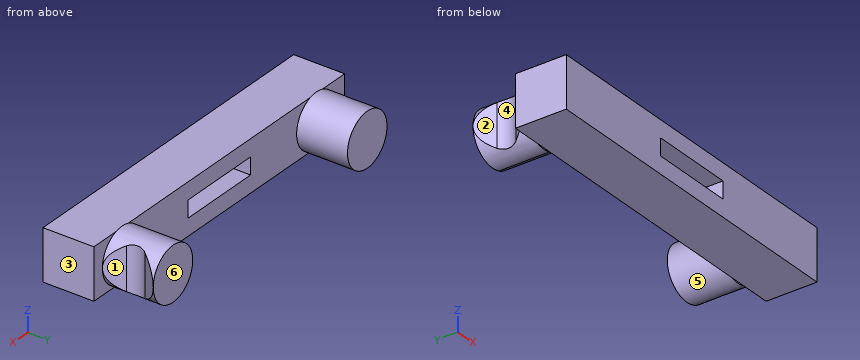
from build123d import *
from build123d.topology import SkipClean

# Parameters (mm, degrees)
SKETCH1_W            = 50.8
SKETCH1_H            = 7.62
BOSS_EXTRUDE1_DEPTH  = 7.62
SKETCH2_W            = 12.7
SKETCH2_H            = 2.54
CUT_EXTRUDE1_DEPTH   = 27.790679349
SKETCH3_R            = 4
BOSS_EXTRUDE2_DEPTH  = 7.62
CUT_EXTRUDE2_DEPTH   = 7.62
FILLET1_R            = 2.54
FILLET1_OF_MIRROR1_R = 2.54


with BuildPart() as part:
    # Sketch1 → Boss-Extrude1 (new body)
    with BuildSketch(Plane(origin=(0, 0, 0), x_dir=(1, 0, 0), z_dir=(0, 1, 0))):
        Rectangle(SKETCH1_W, SKETCH1_H)
    extrude(amount=BOSS_EXTRUDE1_DEPTH)

    # Sketch2 → Cut-Extrude1 (cut, through all)
    with BuildSketch(Plane(origin=(0, 7.62, 0), x_dir=(1, 0, 0), z_dir=(0, 1, 0))):
        Rectangle(SKETCH2_W, SKETCH2_H)
    extrude(amount=-CUT_EXTRUDE1_DEPTH, mode=Mode.SUBTRACT)

    # Sketch3 → Boss-Extrude2 (add)
    with BuildSketch(Plane(origin=(0, 7.62, 0), x_dir=(1, 0, 0), z_dir=(0, 1, 0))):
        with Locations(Location((-19.681240592, 0, 0), (0, 0, 72.269593739))):
            Circle(SKETCH3_R)
    boss_extrude2 = extrude(amount=BOSS_EXTRUDE2_DEPTH)

    # Sketch4 → Cut-Extrude2 (cut, symmetric)
    with SkipClean():  # the faces are left unmerged after this step: merging them gives an invalid solid
        with BuildSketch(Plane.XY):
            Polygon((-23.681240592, 15.24), (-23.681240592, 7.62), (-21.141240592, 11.43), align=None)
        cut_extrude2 = extrude(amount=CUT_EXTRUDE2_DEPTH, both=True, mode=Mode.SUBTRACT)

    # Fillet1
    fillet1_edges = [part.edges().sort_by_distance(p)[0] for p in [
        (-21.141240592, 11.43, 0),
    ]]
    fillet(fillet1_edges, radius=FILLET1_R)

    # Mirror1: Boss-Extrude2, Cut-Extrude2 across plane
    add(boss_extrude2.mirror(Plane(origin=(0, 0, 0), x_dir=(0, 0, 1), z_dir=(1, 0, 0))))
    add(cut_extrude2.mirror(Plane(origin=(0, 0, 0), x_dir=(0, 0, 1), z_dir=(1, 0, 0))), mode=Mode.SUBTRACT)

    # Fillet1 of Mirror1
    fillet1_of_mirror1_edges = [part.edges().sort_by_distance(p)[0] for p in [
        (21.141240592, 11.43, 0),
    ]]
    fillet(fillet1_of_mirror1_edges, radius=FILLET1_OF_MIRROR1_R)


solid = part.part
Can you work these out from the model? Positions are in its coordinate system, mm. Face numbers are marked on the shaded views. A direction names the side the tool comes from. Coordinates: 2 decimals unless noted, no trailing zeros. Loops run counter-clockwise (first coordinate to the right, second up) from the corner with the lowest first, then second, coordinate; pieces in that order, holes last. Notation, with made-up numbers: M -15,-31.75 L 5,-31.75 A28 cw 5,1.25 Z; hole C -27,-27.5 d8. An arc over 180 degrees is marked long. Answer as CSV lines item,"result". Start each with the question number.
1. For pin 1 Ø2.5 at (x, z) = (7.5, 2) entering from +Y; pin 2 Ø2 at (x, z) = (-16.5, 2.5) entering from +Y; pin 3 Ø2.5 at (x, y) = (2, 3.5) entering from +Z; pin 4 Ø6 at (x, y) = (-1, 3.5) entering from -Z, each with a flat end and sliding along its axis, tell me the tip position at first contact or that it passes through.
2. Suppose I cut it at C-C, the plane z = 0.5. List the corners of the cut face in (x, y) for me, plus the area to 3 significant figures.
3. Suppose I cut it at B-B, the plane y = 7. List the corners of the cut face in (x, z) for me.
4. Suppose I cut it at A-A, the plane x = -3. List the corners of the cut face in (y, z) for me, plus the area to 3 significant figures.
5. If I drill on probe 1 along Z at (x, y) = (-3, 4.5); probe 2 along X at (y, z) = (3.5, -0.25); probe 3 along Y at (x, z) = (-2, -2.25), over which ranges is the centre line in solid material (lowest first)? Write a range as [from, to].
6. Thinking about a two-plate mould opening in X: for the marked faces 4, 5 and 6, which applies, +X half, -X half, draft (parallel to the pull), parting line (faces both ways), or undercut?
7. Suppose I cut it at D-D, the plane y = 9. List the corners of the cut face in (x, z) for me, plus the area to 3 significant figures.
8. For the marked faces 1, 2 and 3, which set-ups out of +Z, -Z, +X, -X, +Y, -Y let a thin tool reach every point of the face, with its end or its side?
Output:
1,pin 1,"stops at y = 7.62"
1,pin 2,"stops at y = 15.24"
1,pin 3,"stops at z = 3.81"
1,pin 4,"stops at z = -3.81"
2,outline,"M -25.4,0 L -6.35,0 L -6.35,7.62 L -15.71,7.62 L -15.71,15.24 L -23.65,15.24 L -23.65,15.19 L -22.08,12.84 A2.54 cw -22.08,10.02 L -23.65,7.67 L -23.65,7.62 L -25.4,7.62 Z; M 6.35,0 L 25.4,0 L 25.4,7.62 L 23.65,7.62 L 23.65,7.67 L 22.08,10.02 A2.54 cw 22.08,12.84 L 23.65,15.19 L 23.65,15.24 L 15.71,15.24 L 15.71,7.62 L 6.35,7.62 Z"
2,area,"393 mm^2"
3,outline,"M -25.4,-3.81 L 25.4,-3.81 L 25.4,3.81 L -25.4,3.81 Z; hole M -6.35,-1.27 L 6.35,-1.27 L 6.35,1.27 L -6.35,1.27 Z"
4,outline,"M 0,-3.81 L 7.62,-3.81 L 7.62,-1.27 L 0,-1.27 Z; M 0,1.27 L 7.62,1.27 L 7.62,3.81 L 0,3.81 Z"
4,area,"38.7 mm^2"
5,probe 1,"z = [-3.81, -1.27], [1.27, 3.81]"
5,probe 2,"x = [-25.4, -6.35], [6.35, 25.4]"
5,probe 3,"y = [0, 7.62]"
6,face 4,"-X half"
6,face 5,"undercut"
6,face 6,"draft"
7,outline,"M -22.76,-2.55 A4 ccw long -22.76,2.55 Z; M 22.76,-2.55 L 22.76,2.55 A4 ccw long Z"
7,area,"94.1 mm^2"
8,face 1,"+Z, -Z, +X"
8,face 2,"+Z, -Z, -X"
8,face 3,"+Z, -Z, +X, +Y, -Y"
